Autodesk Inventor part; units mm, degrees
ref_plane "YZ Plane" through (0, 0, 0) normal (1, 0, 0) x (0, 1, 0)
ref_plane "XZ Plane" through (0, 0, 0) normal (0, 1, 0) x (-1, 0, 0)
ref_plane "XY Plane" through (0, 0, 0) normal (0, 0, 1) x (1, 0, 0)
sketch "Sketch1" plane through (0, 0, 0) normal (0, 1, 0) x (-1, 0, 0)
  line L0 (0, 0) -> (25, 0)
  line L1 (25, 0) -> (25, -40)
  line L2 (25, -40) -> (0, -40)
  line L3 (0, -40) -> (0, 0)
  line L4 (25, -40) -> (4, -40)
  line L5 (4, -40) -> (4, -4)
  line L6 (4, -4) -> (25, -4)
  line L7 (25, -4) -> (25, -40)
  point P0 (25, -4)
  dimension "d0" = 4
  dimension "d1" = 4
  dimension "d2" = 40
  dimension "d3" = 25
extrude "Extrusion1" add sketch "Sketch1" along normal blind 100 contours L0 L1 L6 L5 L2 L3
sketch "Sketch2" plane through (0, 100, 0) normal (0, 1, 0) x (1, 0, 0)
  line L0 (0, 0) -> (0, 40)
  line L1 (0, 40) -> (-4, 40)
  line L2 (-4, 40) -> (-4, 4)
  line L3 (-4, 4) -> (-25, 4)
  line L4 (-25, 4) -> (-25, 0)
  line L5 (-25, 0) -> (0, 0)
  line L6 (-25, 0) -> (0, 0)
  line L7 (-17.8564, 0) -> (0, 30.9282)
  line L8 (0, 0) -> (0, 40)
  line L9 (0, 32.9282) -> (-19.0111, 0)
  line L10 (-4, 40) -> (-4, 4)
  point P0 (-16.7017, 4)
  point P1 (-19.0111, 0)
  point P2 (-17.8564, 0)
  point P3 (-15.547, 4)
  point P4 (0, 32.9282)
  point P5 (-4, 26)
  point P6 (-4, 24)
  point P7 (0, 30.9282)
  point P8 (-4, 24)
  dimension "d7" = 30
  dimension "d8" = 1
  dimension "d11" = 20
extrude "Extrusion2" cut sketch "Sketch2" against normal blind 80 contours L7 L2 L9 L0 | L5 L9 L3 L7 | L7 L3 L9 L2
sketch "Sketch3" plane through (0, 100, 0) normal (0, 1, 0) x (1, 0, 0)
  line L0 (-19.0111, 0) -> (-16.7017, 4)
  line L1 (-16.7017, 4) -> (-25, 4)
  line L2 (-25, 4) -> (-25, 0)
  line L3 (-25, 0) -> (-19.0111, 0)
  line L4 (-15.547, 4) -> (-17.8564, 0)
  line L5 (-17.8564, 0) -> (0, 0)
  line L6 (0, 0) -> (0, 30.9282)
  line L7 (0, 30.9282) -> (-4, 24)
  line L8 (-4, 24) -> (-4, 4)
  line L9 (-4, 4) -> (-15.547, 4)
  line L10 (-4, 26) -> (0, 32.9282)
  line L11 (0, 32.9282) -> (0, 40)
  line L12 (0, 40) -> (-4, 40)
  line L13 (-4, 40) -> (-4, 26)
  line L14 (-16.7017, 4) -> (-15.547, 4)
  line L15 (-19.0111, 0) -> (-16.7017, 4)
  line L16 (-17.8564, 0) -> (-19.0111, 0)
  line L17 (-15.547, 4) -> (-17.8564, 0)
  line L18 (-4, 24) -> (-4, 26)
  line L19 (0, 30.9282) -> (-4, 24)
  line L20 (0, 32.9282) -> (0, 30.9282)
  line L21 (-4, 26) -> (0, 32.9282)
  point P0 (0, 32.9282)
extrude "Extrusion3" add sketch "Sketch3" along normal blind 40
properties part number "Knife_guide_30deg_20mm"
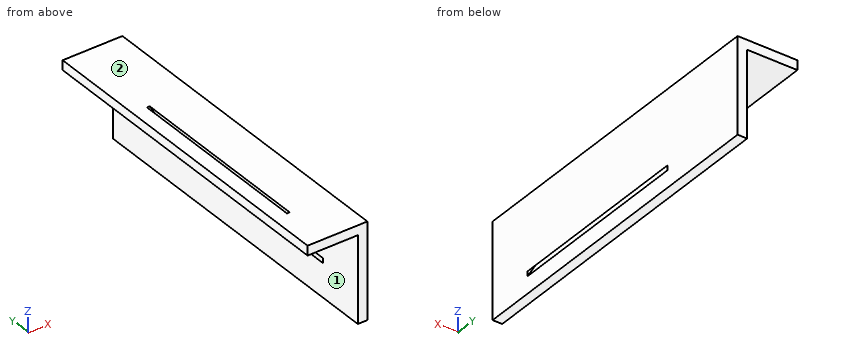
Can you work these out from the model? Positions are in its coordinate system, mm. Face numbers are marked on the shaded views. A direction names the side the tool comes from. Give positions to 0.01 mm unless a question says otherwise; leave off trailing zeros. Order: outer loops, then holes, each group sorted by start corner. A loop starts at its lowest first (then second) coordinate and runs counter-clockwise, first axis right, second up. Notation, with made-up numbers: (9.5, 10.5) - (24.5, 10.5) arc R19 ccw to (24.5, 25.5) - close; hole circle Ø4 at (66.5, 15). An arc over 180 degrees is marked (long way). Write each question's results on one line, items separated by ' | '.
1) Please list where these lines run through material, in increasing order: line 1 along Z through (x, y) = (-13.5, 7.5); line 2 along Y through (x, z) = (-17, -2). Write a range as [from, to].
Final values:
line 1: z = [-4, 0] | line 2: y = [0, 20], [100, 140]
2) Suppose I cut it at A-A, the plane y = 90.5. Write out the boundary of the cut face in (x, z), then the cut area to 3 significant figures.
Final values:
outline: (-25, -4) - (-16.7, -4) - (-19.01, 0) - (-25, 0) - close; (-17.86, 0) - (-15.55, -4) - (-4, -4) - (-4, -24) - (0, -30.93) - (0, 0) - close; (-4, -40) - (0, -40) - (0, -32.93) - (-4, -26) - close | area: 231 mm^2
3) I'm going to push flat-ended pins straight in: pin 1 Ø1 at (x, y) = (-9.5, 53) entering from -Z; pin 2 Ø18 at (y, z) = (57, -15.5) entering from -X. Where does each tip first touch, or does it pass through?
Final values:
pin 1: stops at z = -4 | pin 2: stops at x = -4
4) Suppose I cut it at D-D, the plane z = -7. Write out the boundary of the cut face in (x, y).
Final values:
outline: (-4, 0) - (0, 0) - (0, 140) - (-4, 140) - close
5) Suppose I cut it at B-B, the plane y = 108. Write out the boundary of the cut face in (x, z), then the cut area to 3 significant figures.
Final values:
outline: (-25, -4) - (-4, -4) - (-4, -40) - (0, -40) - (0, 0) - (-25, 0) - close | area: 244 mm^2
6) Suppose I cut it at C-C, the plane z = -28.5. Write out the boundary of the cut face in (x, y), then the cut area to 3 significant figures.
Final values:
outline: (-4, 0) - (0, 0) - (0, 140) - (-4, 140) - close; hole (-2.56, 20) - (-1.4, 20) - (-1.4, 100) - (-2.56, 100) - close | area: 468 mm^2
7) On a 3-axis mill with a long thin cutter (end or side, diameter ignored), from which of +Z, -Z, +X, -X, +Y, -Y can I reach the whole of each face in a straight line? I mean the marked faces 1 and 2. Say none if no direction works.
Final values:
face 1: -Z, -X, +Y, -Y | face 2: +Z, +X, -X, +Y, -Y
